Geometry: final body of the model. Coordinates: model frame, mm. Round coordinates to 2 decimals unless told otherwise and drop trailing zeros. Loops run counter-clockwise (first coordinate to the right, second up) from the corner with the lowest first, then second, coordinate; pieces in that order, holes last. Notation, with made-up numbers: (40.5, 27) -> (65.5, 27) arc R16 cw to (65.5, 41) -> close; hole circle Ø10 at (-37, 55.25). An arc over 180 degrees is marked (long way). Answer in a Markdown table with one row per item.
```python
from build123d import *

# Parameters (mm, degrees)
F1_DEPTH      = 381
F1_DEPTH_BACK = 381
F3_D          = 6.35
F3_DEPTH      = 6.35
F5_D          = 25.4


with BuildPart() as f1:
    # F0 (on Right) → F1 (new body, two sides)
    with BuildSketch(Plane.YZ) as f1_sk:
        Polygon((-69.85, 38.227), (-69.85, 0), (69.85, 0), (69.85, 38.227), (63.5, 38.227), (63.5, 12.827), (31.75, 12.827), (31.75, 38.227), (-31.75, 38.227), (-31.75, 12.827), (-63.5, 12.827), (-63.5, 38.227), align=None)
    extrude(amount=F1_DEPTH)
    extrude(f1_sk.sketch, amount=-F1_DEPTH_BACK)

    # F3
    with Locations(Plane.XZ.offset(69.85)):
        with Locations((0, 25.527)):
            Hole(F3_D / 2, depth=F3_DEPTH)

    # F5 (through all)
    with Locations(Plane.XY.offset(38.227)):
        with Locations((0, 0)):
            Hole(F5_D / 2)


solid = f1.part
```
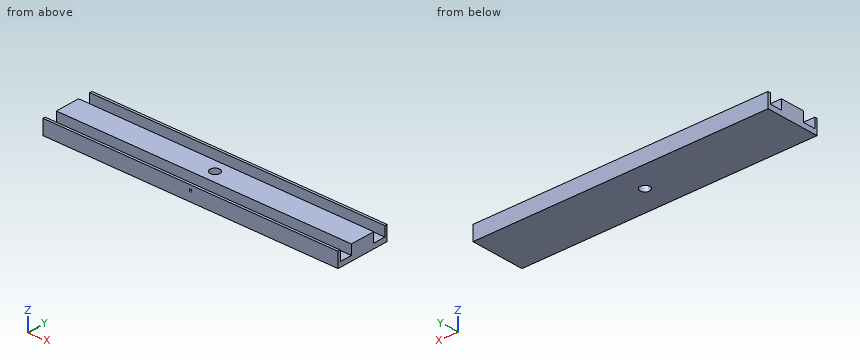
Item 1: Cut plane B-B (x = 226.5). Output: boundary loops of the cut face in (y, z).
Answer:
| item | result |
|---|---|
| outline | (-69.85, 0) -> (69.85, 0) -> (69.85, 38.23) -> (63.5, 38.23) -> (63.5, 12.83) -> (31.75, 12.83) -> (31.75, 38.23) -> (-31.75, 38.23) -> (-31.75, 12.83) -> (-63.5, 12.83) -> (-63.5, 38.23) -> (-69.85, 38.23) -> close |
Item 2: Line query: probe 1 along Y at (x, z) = (0, 13.5); probe 2 along Y at (x, z) = (334.5, 36.5); probe 3 along Y at (x, z) = (0, 26.5). Output: solid intervals per line, ascending. Write a range as [from, to].
Answer:
| item | result |
|---|---|
| probe 1 | y = [-69.85, -63.5], [-31.75, -12.7], [12.7, 31.75], [63.5, 69.85] |
| probe 2 | y = [-69.85, -63.5], [-31.75, 31.75], [63.5, 69.85] |
| probe 3 | y = [-31.75, -12.7], [12.7, 31.75], [63.5, 69.85] |
Item 3: Pin query (flat end, axial travel): pin 1 Ø10 at (x, y) = (221.5, -35.5) entering from -Z; pin 2 Ø1 at (x, y) = (-157, -55.5) entering from +Z. Return the tip coordinate at first contact, or that it passes through.
Answer:
| item | result |
|---|---|
| pin 1 | stops at z = 0 |
| pin 2 | stops at z = 12.83 |
Item 4: Cut plane A-A (y = 0). Output: boundary loops of the cut face in (x, z), then the cut area to 3 significant figures.
Answer:
| item | result |
|---|---|
| outline | (-381, 0) -> (-12.7, 0) -> (-12.7, 38.23) -> (-381, 38.23) -> close; (12.7, 0) -> (381, 0) -> (381, 38.23) -> (12.7, 38.23) -> close |
| area | 28,200 mm² |
Item 5: Cut plane C-C (y = -49). Output: boundary loops of the cut face in (x, z), then the cut area to 3 significant figures.
Answer:
| item | result |
|---|---|
| outline | (-381, 0) -> (381, 0) -> (381, 12.83) -> (-381, 12.83) -> close |
| area | 9,770 mm² |
